Can you work these out from the model? Positions are in its coordinate system, mm. Face numbers are marked on the shaded views. A direction names the side the tool comes from. Give positions to 0.01 mm unless a question says otherwise; leave off trailing zeros. Loops run counter-clockwise (first coordinate to the right, second up) from the corner with the lowest first, then second, coordinate; pieces in that order, holes last.
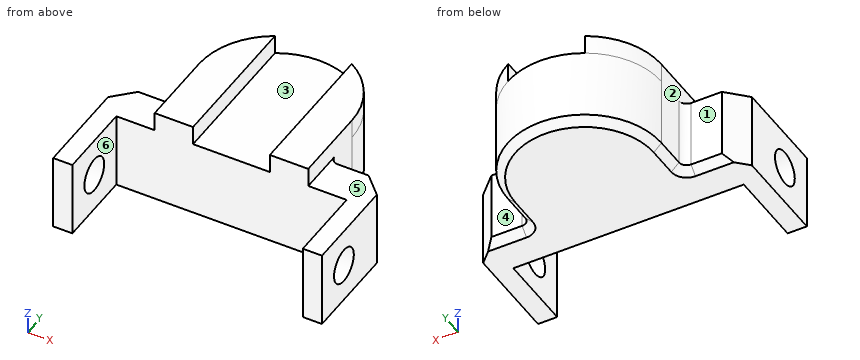
from build123d import *

# Parameters (mm, degrees)
EXTRUDE_1_DEPTH     = 10
SKETCH_2_R          = 4.5
CUT_EXTRUDE_1_DEPTH = 71
CHAMFER_3_SIZE      = 5
FILLET_2_R          = 2
CHAMFER_5_SIZE      = 2
EXTRUDE_2_DEPTH     = 5


with BuildPart() as part:
    # 草图1 → 凸台-拉伸1 (new body, symmetric)
    with BuildSketch(Plane.XY):
        with BuildLine():
            Line((-30, 0), (30, 0))
            Line((30, 0), (30, -20))
            Line((30, -20), (35, -20))
            Line((35, -20), (35, 10))
            Line((35, 10), (20, 10))
            Line((20, 10), (20, 20))
            ThreePointArc((20, 20), (0, 40), (-20, 20))
            Line((-20, 20), (-20, 10))
            Line((-20, 10), (-35, 10))
            Line((-35, 10), (-35, -20))
            Line((-35, -20), (-30, -20))
            Line((-30, -20), (-30, 0))
        make_face()
    extrude(amount=EXTRUDE_1_DEPTH, both=True)

    # 草图2 → 切除-拉伸1 (cut, through all)
    with BuildSketch(Plane.ZY.offset(35)):
        with Locations((0, -10)):
            Circle(SKETCH_2_R)
    extrude(amount=-CUT_EXTRUDE_1_DEPTH, mode=Mode.SUBTRACT)

    # 倒角3
    chamfer_3_edges = [part.edges().sort_by_distance(p)[0] for p in [
        (35, 10, 0),
        (-35, 10, 0),
    ]]
    chamfer(chamfer_3_edges, length=CHAMFER_3_SIZE)

    # 圆角2
    fillet_2_edges = [part.edges().sort_by_distance(p)[0] for p in [
        (-20, 10, 0),
        (20, 10, 0),
    ]]
    fillet(fillet_2_edges, radius=FILLET_2_R)

    # 倒角5
    chamfer_5_edges = [part.edges().sort_by_distance(p)[0] for p in [
        (-20, 16, -10),
        (0, 40, -10),
        (26, 10, -10),
        (-26, 10, -10),
        (20, 16, -10),
        (-20.585786438, 10.585786438, -10),
        (20.585786438, 10.585786438, -10),
    ]]
    chamfer(chamfer_5_edges, length=CHAMFER_5_SIZE)

    # 草图3 → 凸台-拉伸2 (add)
    with BuildSketch(Plane.XY.offset(10)):
        with BuildLine():
            Line((20, 0), (10, 0))
            Line((10, 0), (10, 37.320508076))
            ThreePointArc((10, 37.320508076), (17.320508076, 30), (20, 20))
            Line((20, 20), (20, 0))
        make_face()
        with BuildLine():
            Line((-10, 0), (-10, 37.320508076))
            ThreePointArc((-10, 37.320508076), (-17.320508076, 30), (-20, 20))
            Line((-20, 20), (-20, 0))
            Line((-20, 0), (-10, 0))
        make_face()
    extrude(amount=EXTRUDE_2_DEPTH)


solid = part.part
(1) Suppose I cut it at C-C on z = 13. List the corners of the cut face in (x, y) for me, plus the area to 3 significant figures.
Returned:
outline: (-20, 0) - (-10, 0) - (-10, 37.32) arc R20 ccw to (-20, 20) - close; (10, 0) - (20, 0) - (20, 20) arc R20 ccw to (10, 37.32) - close
area: 646 mm2
(2) Thinking about a two-plate mould opening in X: for the marked faces 1, 2 and 3, which applies, pulls with the +X half, pulls with the -X half, needs draft (parallel to the pull), parting line crosses it, or undercut?
Returned:
face 1: needs draft
face 2: pulls with the -X half
face 3: undercut
(3) Please list where these lines run through material, in increasing order: probe 1 along X at (y, z) = (-16, 2); probe 2 along Z at (x, y) = (-1, 30); probe 3 along Y at (x, z) = (31.3, 0).
Returned:
probe 1: x = -35 to -30, 30 to 35
probe 2: z = -10 to 10
probe 3: y = -20 to -14.5, -5.5 to 8.7
(4) Will these pins go through, and if not, where does the flat tip stop? P1, Ø2, axis at y = 33, z = 6, coming from the -X side; P2, Ø4, axis at x = -26, z = 2, coming from the +Y side; P3, Ø7, axis at y = -10, z = 0, coming from the -X side; P4, Ø4, axis at x = 7.5, y = 14, coming from the +Z side.
Returned:
P1: stops at x = -16
P2: stops at y = 10
P3: passes through
P4: stops at z = 10
(5) Which directions (+Z, -Z, +X, -X, +Y, -Y) give clear straight access to the entire face, cutting with the end or side of a thin tool? Please do the marked faces 4, 5 and 6.
Returned:
face 4: +Z, -Z, +X, +Y
face 5: +Z, +X, +Y, -Y
face 6: +Z, -Z, -Y
(6) Suppose I cut it at B-B on y = -10. List the corners of the cut face in (x, z) for me, plus the area to 3 significant figures.
Returned:
outline: (-35, -10) - (-30, -10) - (-30, -4.5) - (-35, -4.5) - close; (-35, 4.5) - (-30, 4.5) - (-30, 10) - (-35, 10) - close; (30, -10) - (35, -10) - (35, -4.5) - (30, -4.5) - close; (30, 4.5) - (35, 4.5) - (35, 10) - (30, 10) - close
area: 110 mm2
(7) Suppose I cut it at A-A on z = 0. List the corners of the cut face in (x, y) for me, plus the area to 3 significant figures.
Returned:
outline: (-35, -20) - (-30, -20) - (-30, -14.5) - (-35, -14.5) - close; (-35, -5.5) - (-30, -5.5) - (-30, 0) - (30, 0) - (30, -5.5) - (35, -5.5) - (35, 5) - (30, 10) - (22, 10) arc R2 cw to (20, 12) - (20, 20) arc R20 ccw to (-20, 20) - (-20, 12) arc R2 cw to (-22, 10) - (-30, 10) - (-35, 5) - close; (30, -20) - (35, -20) - (35, -14.5) - (30, -14.5) - close
area: 1,820 mm2
(8) Suppose I cut it at D-D on y = 19. List the corners of the cut face in (x, z) for me.
Returned:
outline: (-20, -8) - (-18, -10) - (18, -10) - (20, -8) - (20, 15) - (10, 15) - (10, 10) - (-10, 10) - (-10, 15) - (-20, 15) - close
